Verification items for the finished model (mm, model axes). Face numbers are marked on the shaded views. A direction names the side the tool comes from. Round coordinates to 2 decimals unless told otherwise and drop trailing zeros. Write each loop counter-clockwise with the first axis right and the second up, starting at its lowest first coordinate (ties: lowest second). Pieces come first, ordered by that corner, then holes. Notation, with made-up numbers: M 5.5,22 L 14.5,22 A17 ccw 14.5,29 Z; hole C -2.75,62 d5. An arc over 180 degrees is marked long. One line per item, written item: value. Start each with the question number.
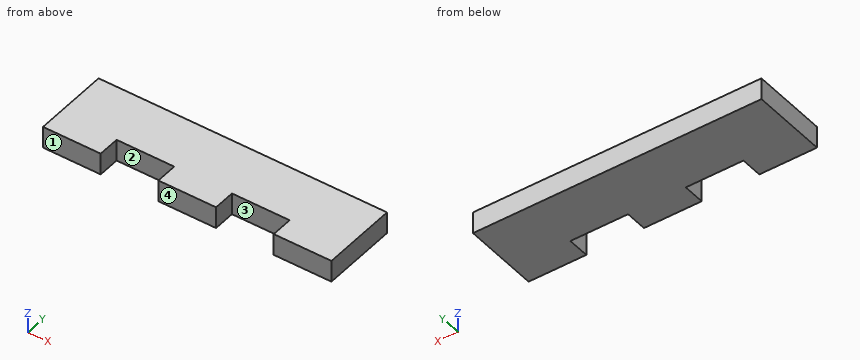
Autodesk Inventor part; units mm, degrees
ref_plane "YZ Plane" through (0, 0, 0) normal (1, 0, 0) x (0, 1, 0)
ref_plane "XZ Plane" through (0, 0, 0) normal (0, 1, 0) x (-1, 0, 0)
ref_plane "XY Plane" through (0, 0, 0) normal (0, 0, 1) x (1, 0, 0)
sketch "Sketch1" plane through (0, 0, 0) normal (0, 0, 1) x (1, 0, 0)
  line L0 (-26.5, 7) -> (26.5, 7)
  line L1 (26.5, 7) -> (26.5, -7)
  line L2 (26.5, -7) -> (-26.5, -7)
  line L3 (-26.5, -7) -> (-26.5, 7)
  line L4 (-26.5, 7) -> (26.5, -7) construction
  line L5 (26.5, 7) -> (-26.5, -7) construction
  line L6 (26.5, -7) -> (15.9, -7)
  line L7 (15.9, -7) -> (15.9, -3)
  line L8 (15.9, -3) -> (26.5, -3)
  line L9 (26.5, -3) -> (26.5, -7)
  line L10 (5.3, -7) -> (5.3, -3)
  line L11 (5.3, -3) -> (15.9, -3)
  line L12 (-5.3, -7) -> (-5.3, -3)
  line L13 (-5.3, -3) -> (5.3, -3)
  line L14 (-15.9, -7) -> (-15.9, -3)
  line L15 (-15.9, -3) -> (-5.3, -3)
  line L16 (-26.5, -7) -> (-26.5, -3)
  line L17 (-26.5, -3) -> (-15.9, -3)
  point P0 (0, 0)
  dimension "d0" = 53
  dimension "d1" = 14
  dimension "d2" = 10.6
  dimension "d3" = 4
  dimension "d6" = 10.6
extrude "Extrusion1" add sketch "Sketch1" along normal blind 4 contours L0 L1 L8 L11 L13 L15 L17 L3 | L17 L14 L2 L3 | L1 L2 L7 L8 | L13 L10 L2 L12
sketch "Sketch2" plane through (0, 0, 4) normal (0, 0, 1) x (1, 0, 0)
  line L0 (-26.5, 7) -> (-26.5, -7)
  line L1 (-26.5, -7) -> (-15.9, -7)
  line L2 (-15.9, -7) -> (-15.9, -3)
  line L3 (-15.9, -3) -> (-5.3, -3)
  line L4 (-5.3, -3) -> (-5.3, -7)
  line L5 (-5.3, -7) -> (5.3, -7)
  line L6 (5.3, -7) -> (5.3, -3)
  line L7 (5.3, -3) -> (15.9, -3)
  line L8 (15.9, -3) -> (15.9, -7)
  line L9 (15.9, -7) -> (26.5, -7)
  line L10 (26.5, -7) -> (26.5, 7)
  line L11 (26.5, 7) -> (-26.5, 7)
  point P0 (0, 0)
equation "\"d1\" = height + e"
equation "\"d2\" = 0.2 * d0"
equation "\"d3\" = e"
equation "\"d6\" = d2"
equation "\"d11\" = e"
equation "\"e\" = 4"
equation "\"height\" = 10"
properties part number "wall1" material "MDF Medium Density Fiberboard"
1) Cross-section at B-B (z = 2.9). Record the boundary of the cut face in (x, y).
2) Cross-section at A-A (y = -3.5). Record the boundary of the cut face in (x, z), then the cut area to 3 significant figures.
3) Access from +Z, -Z, +X, -X, +Y, -Y to the whole of each face (thin tool, end or side, straight path). Record for the marked faces 1 and 2.
4) Thickness scan on line 1 (X direction, y = -3.5, z = 2.25); line 2 (Y direction, x = -10, z = 1.95). Record the ranges inside material, lowest first.
5) Cross-section at C-C (x = -9.5). Record the boundary of the cut face in (y, z), then the cut area to 3 significant figures.
6) Mould release check, pull along X, two halves, no side actions. Record for the marked faces 3 and 4: pulls with the +X half, pulls with the -X half, needs draft (parallel to the pull), parting line crosses it, or undercut.
Results below:
1. outline: M -26.5,-7 L -15.9,-7 L -15.9,-3 L -5.3,-3 L -5.3,-7 L 5.3,-7 L 5.3,-3 L 15.9,-3 L 15.9,-7 L 26.5,-7 L 26.5,7 L -26.5,7 Z
2. outline: M -26.5,0 L -15.9,0 L -15.9,4 L -26.5,4 Z; M -5.3,0 L 5.3,0 L 5.3,4 L -5.3,4 Z; M 15.9,0 L 26.5,0 L 26.5,4 L 15.9,4 Z
2. area: 127 mm²
3. face 1: +Z, -Z, +X, -X, -Y
3. face 2: +Z, -Z, -Y
4. line 1: x = -26.5 to -15.9, -5.3 to 5.3, 15.9 to 26.5
4. line 2: y = -3 to 7
5. outline: M -3,0 L 7,0 L 7,4 L -3,4 Z
5. area: 40.0 mm²
6. face 3: undercut
6. face 4: needs draft
